Model file for the job. Use its own axes, mm. A direction names the side the tool comes from. Coordinates: 2 decimals unless noted, no trailing zeros. Write each loop counter-clockwise with the first axis right and the second up, starting at its lowest first coordinate (ties: lowest second). Pieces come first, ordered by that corner, then holes.
Q1. Drill centre lines: probe 1 along Y at (x, z) = (0, 52); probe 2 along Y at (x, z) = (5, 19.5); probe 3 along X at (y, z) = (1, 21.5). Where is each one in solid material? Low to high.
Q2. Band-saw the part on B-B, the plane z = 8. Write the cut outline in (x, y).
Q3. Pin check, flat tips, straight feed: P1, Ø1.5, axis at x = 4.5, y = 2.5, coming from the +Z side; P2, Ø1.5, axis at x = 1, y = -8, coming from the -Z side; P3, Ø8, axis at y = 6.5, z = 51.5, coming from the -X side; P4, Ø12, axis at y = -3, z = 12.5, coming from the +X side. Stop position of each tip, or through.
Q4. Which spindle directions (+Z, -Z, +X, -X, +Y, -Y) get a long thin tool onto all of the face, cutting with end or side? Do faces 1 (the flat face through (0, 0, 60)), 2 (the cylindrical face through (5.158, 3.955, 23.021)), 3 (the flat face through (2, 8, 4)). Say none if no direction does.
Q5. Band-saw the part on A-A, the plane z = 33. Write the cut outline in (x, y).
from build123d import *

# Parameters (mm, degrees)
REVOLVE_ONTO_SKETCH_ROLL_ANGLE = 90


with BuildPart() as part:
    # Sketch as drawn → Revolve (revolve)
    with BuildSketch(Plane.XY):
        with BuildLine():
            ThreePointArc((-8, 4), (-4.472136, 1.055728), (0, 0))
            Line((0, 60), (0, 0))
            Line((-4, 60), (0, 60))
            Line((-4, 24.5), (-4, 60))
            Line((-6.5, 24.5), (-4, 24.5))
            Line((-6.5, 21.5), (-6.5, 24.5))
            ThreePointArc((-6.5, 21.5), (-10.398317, 17.414815), (-12, 12))
            ThreePointArc((-12, 12), (-16, 8), (-12, 4))
            Line((-8, 4), (-12, 4))
        make_face()
    revolve(axis=Axis((0, 1, 0), (0, 1, 0)))


with BuildPart() as part_1:
    # Revolve onto Sketch roll: moved
    add(part.part.rotate(Axis((0, 0, 0), (1, 0, 0)), REVOLVE_ONTO_SKETCH_ROLL_ANGLE))


with BuildPart() as part_2:
    # Revolve onto Sketch placement: moved
    add(part_1.part)


solid = part_2.part
Answer sheet:
1. probe 1: y = -4 to 4
1. probe 2: y = -7.33 to 7.33
1. probe 3: x = -6.42 to 6.42
2. outline: circle Ø32 at (0, 0)
3. P1: stops at z = 24.5
3. P2: stops at z = 3.18
3. P3: stops at x = -3.12
3. P4: stops at x = 16
4. face 1: +Z, +X, -X, +Y, -Y
4. face 2: +Z
4. face 3: -Z
5. outline: circle Ø8 at (0, 0)
